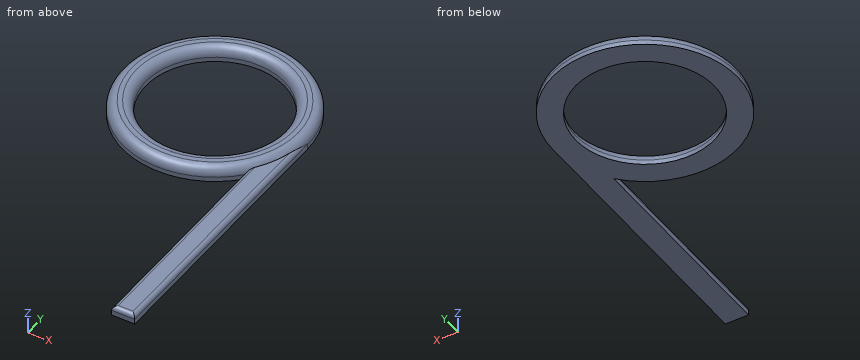
```python
from build123d import *

# Parameters (mm, degrees)
SKETCH_R     = 20
SKETCH_R_2   = 15
PAD_DEPTH    = 3
FILLET_R     = 2
PAD001_DEPTH = 2
FILLET001_R  = 0.9


with BuildPart() as part:
    # Sketch → Pad (new body)
    with BuildSketch(Plane.XY):
        with Locations((-20, 0)):
            Circle(SKETCH_R)
        with Locations((-20, 0)):
            Circle(SKETCH_R_2, mode=Mode.SUBTRACT)
    extrude(amount=PAD_DEPTH)

    # Fillet
    fillet_edges = [part.edges().sort_by_distance(p)[0] for p in [
        (-40, 0, 3),
        (-35, 0, 3),
    ]]
    fillet(fillet_edges, radius=FILLET_R)

    # Sketch001 → Pad001 (join)
    with BuildSketch(Plane.XY):
        Polygon((0, 0), (0, -60), (-5, -60), (-5, -8.660254), align=None)
    extrude(amount=PAD001_DEPTH)

    # Fillet001
    fillet001_edges = [part.edges().sort_by_distance(p)[0] for p in [
        (-5, -36.410028, 2),
        (0, -30, 2),
        (-2.5, -60, 2),
    ]]
    fillet(fillet001_edges, radius=FILLET001_R)


solid = part.part
```
Here's how the part is built. I have some questions about the finished solid (model axes, mm). Coordinates: 2 decimals unless noted, no trailing zeros. Order: outer loops, then holes, each group sorted by start corner. A loop starts at its lowest first (then second) coordinate and runs counter-clockwise, first axis right, second up. Notation, with made-up numbers: M 62.25,26 L 74.25,26 A14 cw 74.25,40 Z; hole C 36.5,-5 d6. An arc over 180 degrees is marked long. Answer as a JSON object with one key per item and string values. Group by question number.
(1) For pin 1 (1.5 mm diameter, centred on x = -20.5, z = 2.5, fed in from -Y); pin 2 (1.2 mm diameter, centred on y = -35, z = 0.5, fed in from -X); pin 3 (1 mm diameter, centred on x = -2.5, y = -37, fed in from +Z), each with a flat end and sliding along its axis, tell me the tip position at first contact or that it passes through.
(2) Suppose I cut it at B-B, the plane y = -39.5. Please give me the cut outline in (x, z), then the cut area to 3 significant figures.
(3) Suppose I cut it at A-A, the plane x = -20. Please give me the cut outline in (y, z), then the cut area to 3 significant figures.
(4) I need wall thicknesses on probe 1 along Y at (x, z) = (-20, 0.35); probe 2 along X at (y, z) = (-47, 1); probe 3 along Y at (x, z) = (-7, 1.85). Which ranges of each line are inside material? Lowest first, please.
Values found:
{
 "1": {"pin 1": "stops at y = -19.85", "pin 2": "stops at x = -5", "pin 3": "stops at z = 2"},
 "2": {"outline": "M -5,0 L 0,0 L 0,1.1 A0.9 ccw -0.9,2 L -4.1,2 A0.9 ccw -5,1.1 Z", "area": "9.65 mm^2"},
 "3": {"outline": "M -20,0 L -15,0 L -15,1 A2 ccw -17,3 L -18,3 A2 ccw -20,1 Z; M 15,0 L 20,0 L 20,1 A2 ccw 18,3 L 17,3 A2 ccw 15,1 Z", "area": "26.6 mm^2"},
 "4": {"probe 1": "y = -20 to -15, 15 to 20", "probe 2": "x = -5 to 0", "probe 3": "y = -14.95 to -7.86, 7.86 to 14.95"}
}
